```python
from build123d import *

# Parameters (mm, degrees)
F1_DEPTH      = 25.4
F3_DEPTH      = 25.4
F5_DEPTH      = 25.4
F5_DEPTH_BACK = 27.94


with BuildPart() as f1:
    # F0 (on Front) → F1 (new body)
    with BuildSketch(Plane.XZ):
        Polygon((43.29247, 51.976606), (-42.395219, 67.168467), (-72.004579, 36.189649), (-83.220236, -32.996144), (-59.443031, -68.303168), (37.460331, -33.151548), align=None)
    extrude(amount=F1_DEPTH)

    # F2 (on Top) → F3 (join)
    with BuildSketch(Plane.XY):
        Polygon((58.817156, 49.181223), (-44.473868, 55.597309), (-44.473868, -53.853892), (40.803842, -62.028117), (66.853315, -40.667363), align=None)
    extrude(amount=F3_DEPTH)

    # F4 (on face) → F5 (join, two sides)
    with BuildSketch(Plane.XY.offset(25.4)) as f5_sk:
        Polygon((-68.057574, 33.107851), (34.036424, 33.107851), (39.893586, 62.429648), (-47.290079, 90.245612), align=None)
    extrude(amount=F5_DEPTH)
    extrude(f5_sk.sketch, amount=-F5_DEPTH_BACK)


solid = f1.part
```
Model file for the job. Use its own axes, mm. A direction names the side the tool comes from. Coordinates: 2 decimals unless noted, no trailing zeros. Order: outer loops, then holes, each group sorted by start corner. A loop starts at its lowest first (then second) coordinate and runs counter-clockwise, first axis right, second up. Notation, with made-up numbers: (10, 70) - (27, 70) arc R22 cw to (27, 78) - close; hole circle Ø4 at (-3.75, -21). An arc over 180 degrees is marked (long way). Return JSON: item names as keys, results as strings. Group by question number.
1) Tool access for faces 4 (the flat face through (-44.474, -39, 13)), 5 (the flat face through (-15, 56, -2.54)), 6 (the flat face through (-44.474, 17, 13)), 7 (the flat face through (-56.99, -12.52, 51.9)): list every direction of +Z, -Z, +X, -X, +Y, -Y with a clear straight run to the whole face (end or side of a thin tool).
2) Mould opens along Y. For faces 1 (the flat face through (37.575, 50.821, 30.43)), 2 (the flat face through (-57.528, 62.077, 24.503)), 3 (the flat face through (38.58, -12.52, -16.81)) say: released by +Y, released by -Y, zero draft, split by the parting line, or undercut.
3) Saw through at C-C, the plane y = 36. Write the cut outline in (x, z).
4) Saw through at A-A, the plane x = 10. Write the cut outline in (y, z).
5) Saw through at B-B, the plane z = 13.5. Write the cut outline in (x, y).
6) Flat gauge pins, fed straight in: P1, Ø10, axis at y = -29, z = -36.5, coming from the +X side; P2, Ø17, axis at x = -34.5, y = 48.5, coming from the -Z side; P3, Ø5, axis at x = -29.5, z = 6.5, coming from the -Y side. Where does each tip first touch, or does it go through?
7) Saw through at D-D, the plane x = 27.5. Write the cut outline in (y, z).
8) Probe line 1 (Z direction, x = 2, y = 41.5); line 2 (Y direction, x = -25, z = -30); line 3 (Z direction, x = -37, y = 8.5). List the from-to ranges inside material, lowest first. Write a range as from..to.
Values found:
{
 "1": {"face 4": "+Z, -Z, -X, -Y", "face 5": "-Z, +X, -X, +Y", "face 6": "+Z, -Z, -X", "face 7": "+Z, -X, -Y"},
 "2": {"face 1": "undercut", "face 2": "released by +Y", "face 3": "zero draft"},
 "3": {"outline": "(-67.01, -2.54) - (34.61, -2.54) - (34.61, 0) - (60, 0) - (60, 25.4) - (34.61, 25.4) - (34.61, 50.8) - (-67.01, 50.8) - close"},
 "4": {"outline": "(-59.08, 0) - (-25.4, 0) - (-25.4, -43.11) - (0, -43.11) - (0, 0) - (33.11, 0) - (33.11, -2.54) - (71.97, -2.54) - (71.97, 50.8) - (33.11, 50.8) - (33.11, 25.4) - (0, 25.4) - (0, 57.88) - (-25.4, 57.88) - (-25.4, 25.4) - (-59.08, 25.4) - close"},
 "5": {"outline": "(-75.68, -25.4) - (-44.47, -25.4) - (-44.47, -53.85) - (40.8, -62.03) - (66.85, -40.67) - (58.82, 49.18) - (37.51, 50.5) - (39.89, 62.43) - (-47.29, 90.25) - (-68.06, 33.11) - (-44.47, 33.11) - (-44.47, 0) - (-75.68, 0) - close"},
 "6": {"P1": "stops at x = 37.47", "P2": "stops at z = -2.54", "P3": "stops at y = -55.53"},
 "7": {"outline": "(-60.75, 0) - (-25.4, 0) - (-25.4, -36.76) - (0, -36.76) - (0, 0) - (33.11, 0) - (33.11, -2.54) - (66.38, -2.54) - (66.38, 50.8) - (33.11, 50.8) - (33.11, 25.4) - (0, 25.4) - (0, 54.78) - (-25.4, 54.78) - (-25.4, 25.4) - (-60.75, 25.4) - close"},
 "8": {"line 1": "z = -2.54..50.8", "line 2": "y = -25.4..0", "line 3": "z = 0..25.4"}
}
